Part model, mm, in its own coordinate system. A direction names the side the tool comes from. Coordinates: 2 decimals unless noted, no trailing zeros. Loops run counter-clockwise (first coordinate to the right, second up) from the corner with the lowest first, then second, coordinate; pieces in that order, holes last. Notation, with made-up numbers: (-12, 18.5) - (28, 18.5) arc R23 ccw to (28, 34.5) - close; hole circle Ø10 at (-26, 2.5). An arc over 180 degrees is marked (long way). Use a Markdown table: item, result. Add a question column.
1. Band-saw the part on A-A, the plane x = -9. Give the cut face in (y, z), plus the area to 3 significant figures.
2. Band-saw the part on D-D, the plane z = -23.5. Give the cut face in (x, y), plus the area to 3 significant figures.
3. Band-saw the part on B-B, the plane y = -1. Give the cut face in (x, z).
4. 3-axis set-ups, long thin cutter, end or side, ignore diameter. For faces 1 (the cylindrical face through (-19.73, 0.87, 14.79)), 2 (the flat face through (9, 9, 30)), 3 (the flat face through (-11.5, -10.8, -10)): which of +Z, -Z, +X, -X, +Y, -Y reach the whole face in a straight line?
5. Pull direction X, two halves, no side cores. Call faces 4 (the flat face through (-12, -5, -66)), 5 (the cylindrical face through (-2.018, 15.368, -37.608)): pulls with the +X half, pulls with the -X half, needs draft (parallel to the pull), parting line crosses it, or undercut.
6. Drop flat-ended pins along their axis: pin 1 (12 mm diameter, centred on x = 16, z = -29, fed in from +Y); pin 2 (1 mm diameter, centred on y = -9, z = -33.5, fed in from -X); pin 3 (2 mm diameter, centred on x = -16, y = -13, fed in from -Z). Give the stop position or say it passes through.
7. Band-saw the part on C-C, the plane z = 12.5. Give the cut face in (x, y).
8. Wall check: probe 1 along Y at (x, z) = (0, -49.5); probe 2 along Y at (x, z) = (0, 16.25); probe 3 along X at (y, z) = (-6, -6.5). Give the ranges that are in metal, low to high. Write a range as [from, to].
from build123d import *

# Parameters (mm, degrees)
F1_DEPTH = 30
F2_R     = 15.5
F2_R_2   = 12.25
F3_DEPTH = 66
F5_DEPTH = 10


# Not quite as in the source:
# - a feature names something its author has since deleted; it is built from what else it names


with BuildPart() as f1:
    # F0 (on Top) → F1 (new body)
    with BuildSketch(Plane.XY):
        with BuildLine():
            ThreePointArc((-19.75, 0), (0, -19.75), (19.75, 0))
            ThreePointArc((19.75, 0), (0, 19.75), (-19.75, 0))
        make_face()
        with BuildLine():
            ThreePointArc((12.25, 0), (0, -12.25), (-12.25, 0))
            ThreePointArc((-12.25, 0), (0, 12.25), (12.25, 0))
        make_face(mode=Mode.SUBTRACT)
    extrude(amount=F1_DEPTH)

    # F2 (on Top) → F3 (join)
    with BuildSketch(Plane.XY):
        Circle(F2_R)
        Circle(F2_R_2, mode=Mode.SUBTRACT)
    extrude(amount=-F3_DEPTH)

    # F4 (on Top) → F5 (join)
    with BuildSketch(Plane.XY):
        with BuildLine():
            ThreePointArc((0, -25), (17.6776695297, -17.6776695297), (25, 0))
            ThreePointArc((25, 0), (-17.6776695297, 17.6776695297), (0, -25))
        make_face()
        with BuildLine():
            ThreePointArc((12.25, 0), (8.6620580695, -8.6620580695), (0, -12.25))
            ThreePointArc((0, -12.25), (-8.6620580695, 8.6620580695), (12.25, 0))
        make_face(mode=Mode.SUBTRACT)
    extrude(amount=-F5_DEPTH)


solid = f1.part
Geometry check:
| question | item | result |
|---|---|---|
| 1 | outline | (-23.32, -10) - (-12.62, -10) - (-12.62, -66) - (-8.31, -66) - (-8.31, 30) - (-17.58, 30) - (-17.58, 0) - (-23.32, 0) - close; (8.31, -66) - (12.62, -66) - (12.62, -10) - (23.32, -10) - (23.32, 0) - (17.58, 0) - (17.58, 30) - (8.31, 30) - close |
| 1 | area | 1,340 mm^2 |
| 2 | outline | circle Ø31 at (0, 0); hole circle Ø24.5 at (0, 0) |
| 2 | area | 283 mm^2 |
| 3 | outline | (-24.98, -10) - (-15.47, -10) - (-15.47, -66) - (-12.21, -66) - (-12.21, 30) - (-19.72, 30) - (-19.72, 0) - (-24.98, 0) - close; (12.21, -66) - (15.47, -66) - (15.47, -10) - (24.98, -10) - (24.98, 0) - (19.72, 0) - (19.72, 30) - (12.21, 30) - close |
| 4 | face 1 | +Z |
| 4 | face 2 | +Z, +X, -X, +Y, -Y |
| 4 | face 3 | -Z |
| 5 | face 4 | needs draft |
| 5 | face 5 | parting line crosses it |
| 6 | pin 1 | stops at y = 11.84 |
| 6 | pin 2 | stops at x = -12.96 |
| 6 | pin 3 | stops at z = -10 |
| 7 | outline | circle Ø39.5 at (0, 0); hole circle Ø24.5 at (0, 0) |
| 8 | probe 1 | y = [-15.5, -12.25], [12.25, 15.5] |
| 8 | probe 2 | y = [-19.75, -12.25], [12.25, 19.75] |
| 8 | probe 3 | x = [-24.27, -10.68], [10.68, 24.27] |
